from build123d import *

# Parameters (mm, degrees)
SKETCH1_R           = 1.778
SKETCH1_R_2         = 4.953
SKETCH1_R_3         = 15.875
BOSS_EXTRUDE1_DEPTH = 1.905


with BuildPart() as part:
    # Sketch1 → Boss-Extrude1 (new body)
    with BuildSketch(Plane.XY):
        with BuildLine():
            ThreePointArc((-133.362998698, -4.004910313), (0, -59.943777505), (133.362998698, -4.004910313))
            ThreePointArc((133.362998698, -4.004910313), (133.290910313, 4.076998698), (125.209001302, 4.004910313))
            ThreePointArc((125.209001302, 4.004910313), (113.793114712, -6.627142221), (101.478252071, -16.203528066))
            ThreePointArc((101.478252071, -16.203528066), (44.101918402, -20.793056649), (12.689537579, 27.439398908))
            ThreePointArc((12.689537579, 27.439398908), (0, 39.624), (-12.689537579, 27.439398908))
            ThreePointArc((-12.689537579, 27.439398908), (-44.101918402, -20.793056649), (-101.478252071, -16.203528066))
            ThreePointArc((-101.478252071, -16.203528066), (-113.793114712, -6.627142221), (-125.209001302, 4.004910313))
            ThreePointArc((-125.209001302, 4.004910313), (-133.290910313, 4.076998698), (-133.362998698, -4.004910313))
        make_face()
        with Locations(Location((0, 0, 0), (0, 0, 180))):
            Circle(SKETCH1_R, mode=Mode.SUBTRACT)
        with Locations(Location((129.286, 0, 0), (0, 0, 180))):
            Circle(SKETCH1_R, mode=Mode.SUBTRACT)
        with Locations(Location((-129.286, 0, 0), (0, 0, 180))):
            Circle(SKETCH1_R, mode=Mode.SUBTRACT)
        with Locations(Location((0, 26.924, 0), (0, 0, 180))):
            Circle(SKETCH1_R_2, mode=Mode.SUBTRACT)
        with Locations(Location((0, -31.75, 0), (0, 0, 180))):
            Circle(SKETCH1_R_3, mode=Mode.SUBTRACT)
    extrude(amount=BOSS_EXTRUDE1_DEPTH)


solid = part.part
The listing builds one solid part. Answer for the finished solid, in the listing's coordinates (mm). A direction names the side the tool comes from. Coordinates: 2 decimals unless noted, no trailing zeros. Order: outer loops, then holes, each group sorted by start corner. A loop starts at its lowest first (then second) coordinate and runs counter-clockwise, first axis right, second up. Notation, with made-up numbers: M -18.5,71.5 L 5.5,71.5 A24 cw 5.5,98.5 Z; hole C 67.5,79.25 d5. An arc over 180 degrees is marked long. Use CSV: the item, a comma, the result in double quotes.
Q1. Determine the mould class of faces 1 (the cylindrical face through (44.86, -21.16, 0.94)), 2 (the flat face through (-11, -17, 1.905)), 3 (the cylindrical face through (0.27, 39.62, 0.94)) for opening direction X: pulls with the +X half, pulls with the -X half, needs draft (parallel to the pull), parting line crosses it, or undercut.
Here are the results:
face 1,"undercut"
face 2,"needs draft"
face 3,"parting line crosses it"
Q2. A tool of negligible diameter and unlimited length cuts with its end or side. For faces 4 (the cylindrical face through (113.959, -6.485, 0.939)), 5 (the cylindrical face through (-2.079, -59.932, 0.939)), from which of +Z, -Z, +X, -X, +Y, -Y can it reach the whole face along a straight path? Write none if from no direction.
Here are the results:
face 4,"+Z, -Z, +Y"
face 5,"+Z, -Z, -Y"
Q3. Section A-A (y = -31.75) is taken. Determine the outline of the cut face in (x, z) (3 decimals).
Here are the results:
outline,"M -98.724,0 L -15.875,0 L -15.875,1.905 L -98.724,1.905 Z; M 15.875,0 L 98.724,0 L 98.724,1.905 L 15.875,1.905 Z"
Q4. Section D-D (y = 11) is taken. Determine the outline of the cut face in (x, z) (1 decimal), then the cut area to 3 significant figures.
Here are the results:
outline,"M -15.8,0 L 15.8,0 L 15.8,1.9 L -15.8,1.9 Z"
area,"60.4 mm2"
Q5. Straight lines are drawn through the part: L1, parallel to Y at x = 0, z = 0.75 (3 decimals); L2, parallel to X at y = -19, z = 0.95; L3, parallel to X at y = -20, z = 1.1. For each, find the intervals that lie inside material, in ascending order.
Here are the results:
L1,"-59.944 to -47.625, -15.875 to -1.778, 1.778 to 21.971, 31.877 to 39.624"
L2,"-116.76 to -97.12, -40.75 to -9.46, 9.46 to 40.75, 97.12 to 116.76"
L3,"-115.49 to -95.32, -42.55 to -10.67, 10.67 to 42.55, 95.32 to 115.49"
Q6. Section C-C (x = -33) is taken. Determine the outline of the cut face in (y, z) (3 decimals), then the cut area to 3 significant figures.
Here are the results:
outline,"M -57.008,0 L -13.605,0 L -13.605,1.905 L -57.008,1.905 Z"
area,"82.7 mm2"
Q7. Section B-B (z = 0.4) is taken. Determine the outline of the cut face in (x, y) (3 decimals), then the cut area to 3 significant figures.
Here are the results:
outline,"M -133.363,-4.005 A186.944 ccw 133.363,-4.005 A5.715 ccw 125.209,4.005 A175.514 cw 101.478,-16.204 A56.29 cw 12.69,27.439 A12.7 ccw -12.69,27.439 A56.29 cw -101.478,-16.204 A175.514 cw -125.209,4.005 A5.715 ccw Z; hole C -129.286,0 d3.556; hole C 0,-31.75 d31.75; hole C 0,26.924 d9.906; hole C 0,0 d3.556; hole C 129.286,0 d3.556"
area,"8,030 mm2"
Q8. Given pin 1 Ø3 at (x, y) = (-129.286, 0) entering from -Z, flat-ended and moving along its own axis, determine where the tip first touches the part or whether it passes through.
Here are the results:
pin 1,"through"
